Input: dimensioned drawing with shaded views. Units: mm. Origin: part minimum x, y, z. A direction names the side the tool comes from. Coordinates: 2 decimals unless noted, no trailing zeros. Loops run counter-clockwise (first coordinate to the right, second up) from the corner with the lowest first, then second, coordinate; pieces in that order, holes last.
Item 1: Section C-C on z = 7. Return loops of the section in (x, y).
Item 2: Section B-B on y = 27.5. Return loops of the section in (x, z), and give its area (3 significant figures).
Item 3: Ray query, line 1 along Y through (x, z) = (5.5, 3.4); line 2 along X through (y, z) = (21.5, 4.75); line 3 along Y through (x, z) = (13.25, 8.25). Return the intervals inside material, ascending.
Item 4: Section D-D on y = 16. Return loops of the section in (x, z).
Item 5: Pull-direction query (Y, two-part tool) for the marked faces 1, 2 and 3; classes: released by +Y, released by -Y, zero draft, split by the parting line, or undercut.
Item 6: Contact query for flat-ended pins moving along their axis: P1, Ø5, axis at x = 7, y = 21.5, coming from the +Z side; P2, Ø4, axis at x = 5.5, y = 48, coming from the +Z side; P3, Ø11, axis at y = 21, z = 14.5, coming from the -X side. Output: stop coordinate, or through.
Item 7: Section A-A on x = 3. Return loops of the section in (y, z).
Item 8: Reachability of the marked faces 4, 5, 6 and 7 from +Z, -Z, +X, -X, +Y, -Y: full face, straight path, thin tool, end or side. Return the list, or none.
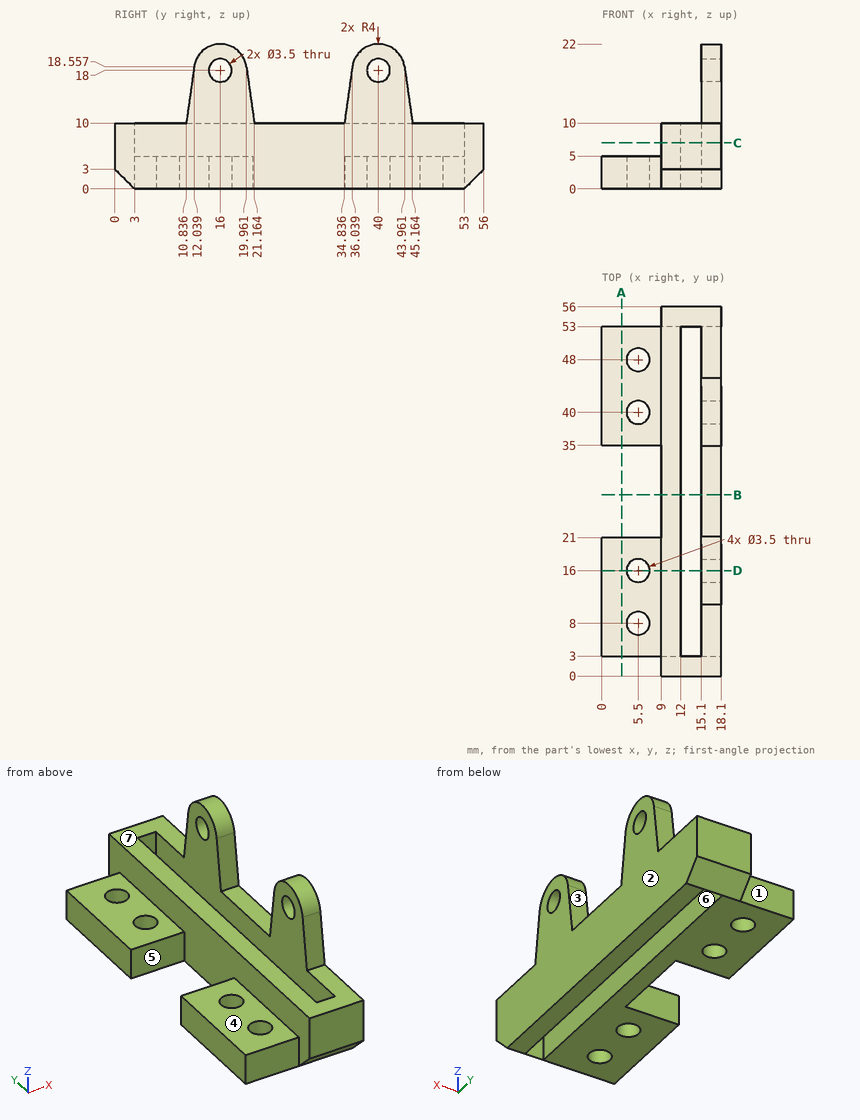
Results found:
1. outline: (9, 0) - (18.1, 0) - (18.1, 56) - (9, 56) - close; hole (12, 3) - (15.1, 3) - (15.1, 53) - (12, 53) - close
2. outline: (9, 0) - (12, 0) - (12, 10) - (9, 10) - close; (15.1, 0) - (18.1, 0) - (18.1, 10) - (15.1, 10) - close
2. area: 60.0 mm2
3. line 1: y = 3 to 6.25, 9.75 to 14.25, 17.75 to 21, 35 to 38.25, 41.75 to 46.25, 49.75 to 53
3. line 2: x = 9 to 12, 15.1 to 18.1
3. line 3: y = 0 to 3, 53 to 56
4. outline: (0, 0) - (3.75, 0) - (3.75, 5) - (0, 5) - close; (7.25, 0) - (12, 0) - (12, 10) - (9, 10) - (9, 5) - (7.25, 5) - close; (15.1, 0) - (18.1, 0) - (18.1, 16.25) - (15.1, 16.25) - close; (15.1, 19.75) - (18.1, 19.75) - (18.1, 22) - (15.1, 22) - close
5. face 1: released by +Y
5. face 2: zero draft
5. face 3: undercut
6. P1: stops at z = 10
6. P2: stops at z = 5
6. P3: stops at x = 9
7. outline: (3, 0) - (21, 0) - (21, 5) - (3, 5) - close; (35, 0) - (53, 0) - (53, 5) - (35, 5) - close
8. face 4: +Z, -X, +Y, -Y
8. face 5: +Z, -Z, -X
8. face 6: +Z, -Z
8. face 7: +Z, -X
